from build123d import *

# Parameters (mm, degrees)
CROQUIS1_W              = 800
CROQUIS1_H              = 900
SALIENTE_EXTRUIR1_DEPTH = 2113
VACIADO2_T              = -10
CROQUIS2_W              = 780
CROQUIS2_H              = 2093
SALIENTE_EXTRUIR2_DEPTH = 5
CORTAR_EXTRUIR1_DEPTH   = 2
SALIENTE_EXTRUIR3_DEPTH = 120


with BuildPart() as part:
    # Croquis1 → Saliente-Extruir1 (new body)
    with BuildSketch(Plane(origin=(0, 0, 0), x_dir=(1, 0, 0), z_dir=(0, 1, 0))):
        Rectangle(CROQUIS1_W, CROQUIS1_H)
    extrude(amount=SALIENTE_EXTRUIR1_DEPTH)

    # Vaciado2
    vaciado2_openings = [part.faces().sort_by_distance(p)[0] for p in [
        (0, 1056.5, 450),
    ]]
    offset(amount=VACIADO2_T, openings=vaciado2_openings, kind=Kind.INTERSECTION)

    # Croquis2 → Saliente-Extruir2 (add)
    with BuildSketch(Plane.XY.offset(450)):
        with Locations((0, 1056.5)):
            Rectangle(CROQUIS2_W, CROQUIS2_H)
    extrude(amount=-SALIENTE_EXTRUIR2_DEPTH)

    # Croquis3 → Cortar-Extruir1 (cut)
    with BuildSketch(Plane.XY.offset(450)):
        Polygon((-136.509991439, 890.520139483), (155.469712472, 890.520139483), (9.479860517, 1243.170950701), align=None)
        Polygon((-63.176808732, 920.19459615), (-42.169545822, 1034.041849102), (9.479860517, 1064.169920858), (9.479860517, 1169.411963853), (65.966344659, 1064.169920858), (-12.532301764, 1019.623730372), (-63.176808732, 898.913148296), align=None, mode=Mode.SUBTRACT)
    extrude(amount=-CORTAR_EXTRUIR1_DEPTH, mode=Mode.SUBTRACT)

    # Croquis4 → Saliente-Extruir3 (add)
    with BuildSketch(Plane.XZ):
        with BuildLine():
            Line((-404.35645152, 475), (404.35645152, 475))
            ThreePointArc((404.35645152, 475), (418.953644638, 468.953644638), (425, 454.35645152))
            Line((425, 454.35645152), (425, -454.35645152))
            ThreePointArc((425, -454.35645152), (418.953644638, -468.953644638), (404.35645152, -475))
            Line((404.35645152, -475), (-404.35645152, -475))
            ThreePointArc((-404.35645152, -475), (-418.953644638, -468.953644638), (-425, -454.35645152))
            Line((-425, -454.35645152), (-425, 454.35645152))
            ThreePointArc((-425, 454.35645152), (-418.953644638, 468.953644638), (-404.35645152, 475))
        make_face()
    extrude(amount=SALIENTE_EXTRUIR3_DEPTH)


solid = part.part
Build history of the part. All positions in model axes, mm. A direction names the side the tool comes from. Round coordinates to 2 decimals unless told otherwise and drop trailing zeros. Write each loop counter-clockwise with the first axis right and the second up, starting at its lowest first coordinate (ties: lowest second). Pieces come first, ordered by that corner, then holes. Notation, with made-up numbers: (55, 51) -> (110, 51) arc R5 cw to (110, 59) -> close; hole circle Ø8 at (33.25, 25.25). An arc over 180 degrees is marked (long way). Write item = value, one per line.
(1) Flat gauge pins, fed straight in: pin 1 (4 mm diameter, centred on y = 549.5, z = 10, fed in from -X); pin 2 (4 mm diameter, centred on x = 96, y = 509, fed in from +Z); pin 3 (5 mm diameter, centred on y = 1455, z = -193, fed in from +X). Where does each tip first touch, or does it go through?
Answer:
pin_1 = -400
pin_2 = 450
pin_3 = 400
(2) Band-saw the part on A-A (z = 166). Give the cut face in (x, y), then the cut area to 3 significant figures.
Answer:
outline = (-425, -120) -> (425, -120) -> (425, 0) -> (400, 0) -> (400, 2113) -> (-400, 2113) -> (-400, 0) -> (-425, 0) -> close; hole (-390, 10) -> (390, 10) -> (390, 2103) -> (-390, 2103) -> close
area = 160,000 mm2
(3) Probe L1, parallel to Y at x = -281, z = -46; L2, parallel to Z at x = 37, y = 34.5; L3, parallel to X at y = 811.5, z = -357.5. List the from-to ranges inside material, lowest first.
Answer:
L1 = -120 to 10, 2103 to 2113
L2 = -450 to -440, 445 to 450
L3 = -400 to -390, 390 to 400
(4) Two-plate mould, pull along Y, no slides. Class faces 5 (the face through (37.328, 1117.528, 449.014)), 6 (the face through (-6, 2113, -6)), 7 (the face through (27.27, 1042.21, 449.01)), 8 (the face through (-6, -59, 475)): pulls with the +Y half, pulls with the -Y half, needs draft (parallel to the pull), parting line crosses it, or undercut.
Answer:
face_5 = undercut
face_6 = pulls with the +Y half
face_7 = undercut
face_8 = needs draft
(5) Band-saw the part on C-C (x = -198). Give the cut face in (y, z), then the cut area to 3 significant figures.
Answer:
outline = (-120, -475) -> (0, -475) -> (0, -450) -> (2113, -450) -> (2113, 450) -> (0, 450) -> (0, 475) -> (-120, 475) -> close; hole (10, -440) -> (2103, -440) -> (2103, 445) -> (10, 445) -> close
area = 163,000 mm2
(6) Band-saw the part on B-B (y = 811). Give the cut face in (x, z), then the cut area to 3 significant figures.
Answer:
outline = (-400, -450) -> (400, -450) -> (400, 450) -> (-400, 450) -> close; hole (-390, -440) -> (390, -440) -> (390, 445) -> (-390, 445) -> close
area = 29,700 mm2
(7) Tool access for faces 1 (the face through (-62.5, 1069.3, 449)), 2 (the face through (-94, 1071, 450)), 3 (the face through (-6, 1042, -450)), 4 (the face through (-390, 1042, 9)): list every direction of +Z, -Z, +X, -X, +Y, -Y with a clear straight run to the whole face (end or side of a thin tool).
Answer:
face_1 = +Z
face_2 = +Z, +X, -X, +Y
face_3 = -Z, +X, -X, +Y
face_4 = none
